Autodesk Inventor part; units mm, degrees
ref_plane "YZ Plane" through (0, 0, 0) normal (1, 0, 0) x (0, 1, 0)
ref_plane "XZ Plane" through (0, 0, 0) normal (0, 1, 0) x (-1, 0, 0)
ref_plane "XY Plane" through (0, 0, 0) normal (0, 0, 1) x (1, 0, 0)
sketch "Sketch1" plane through (0, 0, 0) normal (0, 1, 0) x (-1, 0, 0)
  circle A0 centre (0, 0) radius 6.35 construction
  line L0 (6.35, -3.6662) -> (0, -7.3323)
  line L1 (0, -7.3323) -> (-6.35, -3.6662)
  line L2 (-6.35, -3.6662) -> (-6.35, 3.6662)
  line L3 (-6.35, 3.6662) -> (0, 7.3323)
  line L4 (0, 7.3323) -> (6.35, 3.6662)
  line L5 (6.35, 3.6662) -> (6.35, -3.6662)
  circle A1 centre (0, 0) radius 9.525
  point P0 (6.35, 0)
  dimension "d0" = 12.7
  dimension "d1" = 19.05
extrude "Extrusion1" add sketch "Sketch1" along normal blind 6.35
sketch "Sketch2" plane through (0, 6.35, 0) normal (0, 1, 0) x (1, 0, 0)
  line L0 (-6.35, 3.6662) -> (0, 7.3323)
  line L1 (0, 7.3323) -> (6.35, 3.6662)
  line L2 (-6.35, -3.6662) -> (-6.35, 3.6662)
  line L3 (0, -7.3323) -> (-6.35, -3.6662)
  line L4 (6.35, -3.6662) -> (0, -7.3323)
  line L5 (6.35, 3.6662) -> (6.35, -3.6662)
  line L6 (-7.85, 4.5322) -> (0, 9.0644)
  line L7 (0, 9.0644) -> (7.85, 4.5322)
  line L8 (7.85, 4.5322) -> (7.85, -4.5322)
  line L9 (7.85, -4.5322) -> (0, -9.0644)
  line L10 (0, -9.0644) -> (-7.85, -4.5322)
  line L11 (-7.85, -4.5322) -> (-7.85, 4.5322)
  point P0 (0, 0)
  dimension "d4" = 1.5
extrude "Extrusion2" cut sketch "Sketch2" against normal blind 25.4 contours L0 L1 L5 L4 L3 L2 | L6 L7 L8 L9 L10 L11
properties part number "SportGearbox_HexDiffGearSpacer"
Source: CAD feature listing. Evaluate the final solid. Frame: model axes, mm. A direction names the side the tool comes from. Give positions to 0.01 mm unless a question says otherwise; leave off trailing zeros. Write each loop counter-clockwise with the first axis right and the second up, starting at its lowest first coordinate (ties: lowest second). Pieces come first, ordered by that corner, then holes. Notation, with made-up numbers: (69, -24) -> (80, -24) arc R27 ccw to (80, -4) -> close; hole circle Ø1 at (69.25, -28.5). An arc over 180 degrees is marked (long way). Write item = value, one per line.
Q1. Line query: line 1 (X direction, y = 0.5, z = 0.25); line 2 (X direction, y = 3, z = 6.5); line 3 (Z direction, x = 2, y = 5). Output: solid intervals per line, ascending. Write a range as from..to.
Here are the results:
line_1 = -9.52..-7.85, 7.85..9.52
line_2 = -6.96..-4.44, 4.44..6.96
line_3 = -9.31..-7.91, 7.91..9.31
Q2. First-contact query: pin 1 (1.5 mm diameter, centred on x = 4.5, y = 2, fed in from +Z); pin 2 (3 mm diameter, centred on x = -2, y = 3, fed in from -Z); pin 3 (1 mm diameter, centred on y = 3, z = -7, fed in from -X); pin 4 (3 mm diameter, centred on y = 3, z = 1, fed in from +X) (3 decimals). Flat tips, straight axial feed; report the tip coordinate or a pass-through.
Here are the results:
pin_1 = 8.76
pin_2 = -9.51
pin_3 = -6.96
pin_4 = 9.525
Q3. Mould query, pull axis Z, two halves, no side actions, for faces 1 (the face through (7.559, 3.131, 5.796)), 2 (the face through (4, 6.35, -7)), 3 (the face through (-3.87, 3.22, 6.83)). Classes: +Z half, -Z half, draft (parallel to the pull), parting line (faces both ways), or undercut.
Here are the results:
face_1 = parting line
face_2 = draft
face_3 = undercut
Q4. Reachability of faces 4 (the face through (4, 0, -7)), 5 (the face through (3.98, 3.219, 6.767)) from +Z, -Z, +X, -X, +Y, -Y: full face, straight path, thin tool, end or side. Return the list, or none.
Here are the results:
face_4 = +Z, -Z, +X, -X, -Y
face_5 = +Y, -Y
Q5. Cut plane B-B on z = 0. Return loops of the section in (x, y) (3 decimals), then the cut area to 3 significant figures.
Here are the results:
outline = (-9.525, 0) -> (-7.85, 0) -> (-7.85, 6.35) -> (-9.525, 6.35) -> close; (7.85, 0) -> (9.525, 0) -> (9.525, 6.35) -> (7.85, 6.35) -> close
area = 21.3 mm²
Q6. Cut plane C-C on x = 4.5. Return loops of the section in (y, z), then the cut area to 3 significant figures.
Here are the results:
outline = (0, -8.39) -> (6.35, -8.39) -> (6.35, -6.47) -> (0, -6.47) -> close; (0, 6.47) -> (6.35, 6.47) -> (6.35, 8.39) -> (0, 8.39) -> close
area = 24.5 mm²
Q7. Cut plane A-A on y = 3. Return loops of the section in (x, z) (3 decimals), then the cut area to 3 significant figures.
Here are the results:
outline = circle Ø19.05 at (0, 0); hole (-7.85, -4.532) -> (0, -9.064) -> (7.85, -4.532) -> (7.85, 4.532) -> (0, 9.064) -> (-7.85, 4.532) -> close
area = 71.6 mm²
